Autodesk Inventor part; units mm, degrees
ref_plane "YZ Plane" through (0, 0, 0) normal (1, 0, 0) x (0, 1, 0)
ref_plane "XZ Plane" through (0, 0, 0) normal (0, 1, 0) x (-1, 0, 0)
ref_plane "XY Plane" through (0, 0, 0) normal (0, 0, 1) x (1, 0, 0)
sketch "Sketch1" plane through (0, 0, 0) normal (0, 1, 0) x (-1, 0, 0)
  line L0 (53.2003, -37.719) -> (-53.2003, -37.719)
  line L1 (-53.2003, -37.719) -> (-53.2003, 37.719)
  line L2 (-53.2003, 37.719) -> (53.2003, 37.719)
  line L3 (53.2003, 37.719) -> (53.2003, -37.719)
  line L4 (53.2003, -37.719) -> (-53.2003, 37.719) construction
  line L5 (-53.2003, -37.719) -> (53.2003, 37.719) construction
  point P0 (0, 0)
  dimension "d0" = 106.4006
  dimension "d1" = 75.438
extrude "Extrusion1" add sketch "Sketch1" along normal blind 6.35
sketch "Sketch2" plane through (0, 6.35, 0) normal (0, 1, 0) x (1, 0, 0)
  line L0 (53.2003, -37.719) -> (53.2003, 37.719)
  line L1 (53.2003, -37.719) -> (53.2003, -34.544)
  line L2 (53.2003, -34.544) -> (50.0761, -34.544)
  line L3 (53.2003, 37.719) -> (53.2003, 34.544)
  line L4 (53.2003, 34.544) -> (50.0761, 34.544)
  line L5 (50.0761, 34.544) -> (50.0761, -34.544)
  line L6 (53.2003, -34.544) -> (53.2003, 34.544)
  point P0 (0, 0)
  dimension "d4" = 3.175
  dimension "d5" = 3.1242
  dimension "d6" = 3.175
extrude "Extrusion2" add sketch "Sketch2" along normal blind 68.58
fillet "Fillet1" radius 3.175 1 edges at (50.0761, 6.35, 0)
sketch "Sketch3" plane through (0, 0, 0) normal (0, -1, 0) x (1, 0, 0)
  line L0 (-9.525, 8.763) -> (9.525, 8.763)
  line L1 (9.525, 8.763) -> (9.525, -8.763)
  line L2 (9.525, -8.763) -> (-9.525, -8.763)
  line L3 (-9.525, -8.763) -> (-9.525, 8.763)
  line L4 (-9.525, 8.763) -> (9.525, -8.763) construction
  line L5 (9.525, 8.763) -> (-9.525, -8.763) construction
  line L6 (9.525, -8.763) -> (-9.525, -8.763)
  line L7 (-9.525, -8.763) -> (-9.525, -4.699)
  line L8 (-9.525, -4.699) -> (9.525, -4.699)
  line L9 (9.525, -4.699) -> (9.525, -8.763)
  line L10 (9.525, 8.763) -> (-9.525, 8.763)
  line L11 (-9.525, 8.763) -> (-9.525, 4.699)
  line L12 (-9.525, 4.699) -> (9.525, 4.699)
  line L13 (9.525, 4.699) -> (9.525, 8.763)
  point P0 (0, 0)
  dimension "d10" = 19.05
  dimension "d11" = 17.526
  dimension "d12" = 4.064
  dimension "d13" = 4.064
extrude "Extrusion3" cut sketch "Sketch3" against normal blind 68.58 contours L0 L1 L12 L3 | L8 L1 L2 L3
sketch "Sketch4" plane through (0, 0, 0) normal (0, -1, 0) x (1, 0, 0)
  point P0 (0, 0)
sketch "Sketch5" plane through (0, 0, 0) normal (0, -1, 0) x (1, 0, 0)
  point P0 (0, 0)
sketch "Sketch6" plane through (53.2003, 0, -37.719) normal (0, 0, -1) x (-1, 0, 0)
  line L0 (106.4006, 0) -> (0, 0)
  line L1 (0, 6.35) -> (106.4006, 6.35)
  line L2 (106.4006, 0) -> (0, 0)
  line L3 (0, 0) -> (0, 6.35)
  line L4 (0, 6.35) -> (106.4006, 6.35)
  line L5 (106.4006, 6.35) -> (106.4006, 0)
  point P0 (53.2003, 0)
sketch "Sketch7" plane through (0, 6.35, 0) normal (0, 1, 0) x (1, 0, 0)
  line L0 (53.2003, 34.544) -> (53.2003, 37.719)
  line L1 (46.9519, -37.719) -> (53.2003, -37.719)
  line L2 (53.2003, -37.719) -> (53.2003, 37.719)
  line L3 (53.2003, 37.719) -> (46.9519, 37.719)
  line L4 (46.9519, 37.719) -> (46.9519, -37.719)
  line L5 (50.0761, 34.544) -> (50.0761, -34.544)
  line L6 (46.9519, -37.719) -> (53.2003, 37.719) construction
  line L7 (53.2003, -37.719) -> (46.9519, 37.719) construction
  point P0 (0, 0)
  point P1 (50.0761, 0)
extrude "Extrusion4" add sketch "Sketch7" along normal blind 68.58
sketch "Sketch8" plane through (0, 74.93, 0) normal (0, 1, 0) x (1, 0, 0)
  line L0 (53.2003, -37.719) -> (53.2003, 37.719)
  line L1 (53.2003, 37.719) -> (46.9519, 37.719)
  line L2 (53.2003, -37.719) -> (50.0761, -37.719)
  line L3 (50.0761, -37.719) -> (50.0761, 37.719)
  line L4 (50.0761, 37.719) -> (53.2003, 37.719)
  line L5 (53.2003, 37.719) -> (53.2003, -37.719)
  line L6 (46.9519, -37.719) -> (53.2003, -37.719)
  line L7 (50.0761, 37.719) -> (46.9519, 37.719)
  line L8 (46.9519, 37.719) -> (46.9519, -37.719)
  line L9 (46.9519, -37.719) -> (50.0761, -37.719)
  line L10 (50.0761, -37.719) -> (50.0761, 37.719)
  point P0 (0, 0)
extrude "Extrusion5" cut sketch "Sketch8" against normal blind 68.58 contours L6 L8 L1 L3
sketch "Sketch9" plane through (53.2003, 0, -37.719) normal (0, 0, -1) x (-1, 0, 0)
  line L0 (3.1242, 6.35) -> (106.4006, 6.35)
  line L1 (106.4006, 6.35) -> (0, 6.35)
  line L2 (0, 6.35) -> (0, 0)
  line L3 (0, 0) -> (106.4006, 0)
  line L4 (106.4006, 0) -> (106.4006, 6.35)
  point P0 (53.2003, 0)
extrude "Extrusion6" add sketch "Sketch9" along normal blind 5.715
sketch "Sketch10" plane through (-53.2003, 0, 37.719) normal (0, 0, 1) x (1, 0, 0)
  line L0 (0, 6.35) -> (106.4006, 6.35)
  line L1 (106.4006, 0) -> (106.4006, 74.93)
  line L2 (0, 6.35) -> (106.4006, 6.35)
  line L3 (106.4006, 6.35) -> (106.4006, 0)
  line L4 (106.4006, 0) -> (0, 0)
  line L5 (0, 0) -> (0, 6.35)
  point P0 (53.2003, 0)
extrude "Extrusion7" add sketch "Sketch10" along normal blind 5.715
sketch "Sketch11" plane through (-53.2003, 0, -43.434) normal (-1, 0, 0) x (0, 0, 1)
  line L0 (0, 0) -> (0, 6.35)
  line L1 (86.868, 0) -> (0, 0)
  line L2 (0, 6.35) -> (86.868, 6.35)
  line L3 (86.868, 6.35) -> (86.868, 0)
  line L4 (86.868, 0) -> (0, 0)
  line L5 (0, 0) -> (0, 6.35)
  point P0 (43.434, 0)
extrude "Extrusion8" add sketch "Sketch11" along normal blind 5.715
sketch "Sketch12" plane through (53.2003, 0, -43.434) normal (0, 0, -1) x (-1, 0, 0)
  line L0 (0, 6.35) -> (112.1156, 6.35)
  line L1 (0, 6.35) -> (0, 3.81)
  line L2 (0, 0) -> (112.1156, 0)
  line L3 (0, 3.81) -> (0, 6.35)
  point P0 (53.2003, 0)
  dimension "d26" = 2.54
sketch "Sketch13" plane through (0, 0, 0) normal (0, -1, 0) x (1, 0, 0)
  line L0 (-61.9125, -50.8) -> (61.9125, -50.8)
  line L1 (61.9125, -50.8) -> (61.9125, 50.8)
  line L2 (61.9125, 50.8) -> (-61.9125, 50.8)
  line L3 (-61.9125, 50.8) -> (-61.9125, -50.8)
  line L4 (-61.9125, -50.8) -> (61.9125, 50.8) construction
  line L5 (61.9125, -50.8) -> (-61.9125, 50.8) construction
  point P0 (0, 0)
extrude "Extrusion9" cut sketch "Sketch13" against normal blind 3.81
sketch "Sketch14" plane through (53.2003, 6.35, -37.719) normal (1, 0, 0) x (0, 0, -1)
  line L0 (0, 0) -> (0, 68.58)
  line L1 (0, 34.29) -> (-6.35, 34.29)
  line L2 (-6.35, 34.29) -> (0, 34.29)
  line L3 (-33.02, -2.54) -> (-33.02, 0)
  line L4 (-33.02, 0) -> (-33.02, 6.35)
  line L5 (-33.02, 6.35) -> (-33.02, 0)
  line L6 (-33.02, 0) -> (-33.02, 6.35)
  line L7 (-69.088, 62.23) -> (-6.35, 62.23)
  line L8 (-6.35, 62.23) -> (-6.35, 6.35)
  line L9 (-6.35, 6.35) -> (-69.088, 6.35)
  line L10 (-69.088, 6.35) -> (-69.088, 62.23)
  line L11 (-69.088, 62.23) -> (-6.35, 6.35) construction
  line L12 (-6.35, 62.23) -> (-69.088, 6.35) construction
  point P0 (-37.719, -6.35)
  point P1 (-37.719, 34.29)
extrude "Extrusion10" cut sketch "Sketch14" against normal blind 381
properties part number "Boxpt2"
Geometry check sheet. Reference: the model listing, model coordinates, mm. A direction names the side the tool comes from. Coordinates: 2 decimals unless noted, no trailing zeros. Order: outer loops, then holes, each group sorted by start corner. A loop starts at its lowest first (then second) coordinate and runs counter-clockwise, first axis right, second up. Notation, with made-up numbers: (-18.5, 52.25) -> (-2.5, 52.25) arc R21 ccw to (-2.5, 56.25) -> close; hole circle Ø11 at (42.25, 36). An arc over 180 degrees is marked (long way). Use a Markdown table: item, result. Add a question column.
1. Mould release check, pull along Z, two halves, no side actions. Record for faces 4 (the face through (52, 40, 31.369)), 5 (the face through (52, 40, 37.719)), 6 (the face through (53.2, 10, 3)): pulls with the +Z half, pulls with the -Z half, needs draft (parallel to the pull), parting line crosses it, or undercut.
2. Material ranges on L1, parallel to Y at x = 20.5, z = -18.5; L2, parallel to X at y = 71, z = -29.5, recorded low to high.
3. Go/stop test with flat-tipped pins: pin 1 Ø0.9 at (x, y) = (52, 32) entering from +Z; pin 2 Ø3.5 at (x, y) = (51.5, 37) entering from -Z; pin 3 Ø6 at (y, z) = (66.5, -22) entering from -X. Record where each tip stops, or that it passes through.
4. Cross-section at A-A (y = 66.5). Enter the section's corners in (x, z), and give its area (3 significant figures).
5. Set-up check for faces 1 (the face through (50.076, 11, 1)), 2 (the face through (52, 12.7, 0)), 3 (the face through (-9.525, 5, -7)): record each of +Z, -Z, +X, -X, +Y, -Y from which the full face is reachable in a straight line by a thin tool's end or side.
6. Cross-section at C-C (x = 38). Enter the section's corners in (y, z).
Filled sheet:
| question | item | result |
|---|---|---|
| 1 | face 4 | undercut |
| 1 | face 5 | pulls with the +Z half |
| 1 | face 6 | needs draft |
| 2 | L1 | 3.81 to 6.35 |
| 2 | L2 | 50.08 to 53.2 |
| 3 | pin 1 | z = 37.72 |
| 3 | pin 2 | z = -37.72 |
| 3 | pin 3 | x = 50.08 |
| 4 | outline | (50.08, -37.72) -> (53.2, -37.72) -> (53.2, -31.37) -> (50.08, -31.37) -> close; (50.08, 31.37) -> (53.2, 31.37) -> (53.2, 37.72) -> (50.08, 37.72) -> close |
| 4 | area | 39.7 mm2 |
| 5 | face 1 | +Z, -Z, -X, +Y |
| 5 | face 2 | +X, -X |
| 5 | face 3 | +Y, -Y |
| 6 | outline | (3.81, -43.43) -> (6.35, -43.43) -> (6.35, 43.43) -> (3.81, 43.43) -> close |
